Geometry: final body of the model. Coordinates: model frame, mm. A direction names the side the tool comes from. Coordinates: 2 decimals unless noted, no trailing zeros. Loops run counter-clockwise (first coordinate to the right, second up) from the corner with the lowest first, then second, coordinate; pieces in that order, holes last. Notation, with made-up numbers: (23.25, 86.5) - (36.25, 86.5) arc R19 ccw to (36.25, 103.5) - close; hole circle Ø4 at (8, 88). An arc over 180 degrees is marked (long way). Answer in a Markdown table with one row per item.
from build123d import *

# Parameters (mm, degrees)
BASE_FLANGE1_DEPTH         = 3.175
F_4_2_4_2_DIAMETER_HOLE1_D = 4.2
F_3_3_3_3_DIAMETER_HOLE1_D = 3.3
EDGE_FLANGE1_DEPTH         = 38.176085753
EDGE_FLANGE1_START         = 3.175
EDGE_FLANGE1_PROFILE_R     = 1.6
EDGE_FLANGE1_PROFILE_R_2   = 11.5
EDGE_FLANGE1_PROFILE_R_3   = 2.6
EDGE_FLANGE1_FLAT_DEPTH    = 3.175


# Sheet-metal steps are written as plain solids
with BuildPart() as part:
    # Sketch11 → Base-Flange1 (new body)
    with BuildSketch(Plane.XZ.offset(2.7625)):
        with BuildLine():
            Line((36.2, 21.175), (36.2, 15.175))
            ThreePointArc((36.2, 15.175), (30, 8.975), (23.8, 15.175))
            Line((23.8, 15.175), (23.8, 21.175))
            ThreePointArc((23.8, 21.175), (23.214213562, 22.589213562), (21.8, 23.175))
            Line((21.8, 23.175), (-7, 23.175))
            ThreePointArc((-7, 23.175), (-9.121320344, 22.296320344), (-10, 20.175))
            Line((-10, 20.175), (-10, 17.93389))
            ThreePointArc((-10, 17.93389), (-15, 12.93389), (-10, 7.93389))
            Line((-10, 7.93389), (-10, 7.7625))
            ThreePointArc((-10, 7.7625), (-9.121320344, 5.641179656), (-7, 4.7625))
            Line((-7, 4.7625), (67, 4.7625))
            ThreePointArc((67, 4.7625), (69.121320344, 5.641179656), (70, 7.7625))
            Line((70, 7.7625), (70, 7.93389))
            ThreePointArc((70, 7.93389), (75, 12.93389), (70, 17.93389))
            Line((70, 17.93389), (70, 20.175))
            ThreePointArc((70, 20.175), (69.121320344, 22.296320344), (67, 23.175))
            Line((67, 23.175), (38.2, 23.175))
            ThreePointArc((38.2, 23.175), (36.785786438, 22.589213562), (36.2, 21.175))
        make_face()
    extrude(amount=-BASE_FLANGE1_DEPTH)

    # Ø4.2 (4.2) Diameter Hole1 (through all)
    with Locations(Plane(origin=(0, -2.7625, 0), x_dir=(-1, 0, 0), z_dir=(0, -1, 0))):
        with Locations((-70, -12.93389), (10, -12.93389)):
            Hole(F_4_2_4_2_DIAMETER_HOLE1_D / 2)

    # Ø3.3 (3.3) Diameter Hole1 (through all)
    with Locations(Plane(origin=(0, 0.4125, 0), x_dir=(1, 0, 0), z_dir=(0, 1, 0))):
        with Locations((5, -12.93389), (55, -12.93389)):
            Hole(F_3_3_3_3_DIAMETER_HOLE1_D / 2)

    # Edge-Flange1 bend section (across the edge) → Edge-Flange1 (add)
    with BuildSketch(Plane(origin=(44.262809753, 0.4125, 3.175), x_dir=(0, 0, 1), z_dir=(-1, 0, 0))):
        with BuildLine():
            Line((-3.175, 1.5875), (0, 1.5875))
            ThreePointArc((0, 1.5875), (0.464967985, 0.464967985), (1.5875, 0))
            Line((1.5875, 0), (1.5875, -3.175))
            ThreePointArc((1.5875, -3.175), (-1.780096045, -1.780096045), (-3.175, 1.5875))
        make_face()
    extrude(amount=EDGE_FLANGE1_DEPTH)

    # Edge-Flange1 profile (on flange) → Edge-Flange1 flat (add)
    with BuildSketch(Plane(origin=(0, 0.4125, 3.175), x_dir=(-1, 0, 0), z_dir=(0, 0, -1)).offset(EDGE_FLANGE1_START)):
        with BuildLine():
            ThreePointArc((-6.086724, 42.5875), (-6.672510438, 44.001713562), (-8.086724, 44.5875))
            Line((-8.086724, 44.5875), (-42.262809753, 44.5875))
            ThreePointArc((-42.262809753, 44.5875), (-43.677023316, 44.001713562), (-44.262809753, 42.5875))
            Line((-44.262809753, 42.5875), (-44.262809753, 39.575887728))
            ThreePointArc((-44.262809753, 39.575887728), (-46.5, 34.902424049), (-44.262809753, 30.22896037))
            Line((-44.262809753, 30.22896037), (-44.262809753, 1.5875))
            Line((-44.262809753, 1.5875), (-6.086724, 1.5875))
            Line((-6.086724, 1.5875), (-6.086724, 42.5875))
        make_face()
        with Locations((-13.100505063, 10.688005063)):
            Circle(EDGE_FLANGE1_PROFILE_R, mode=Mode.SUBTRACT)
        with Locations((-23, 20.5875)):
            Circle(EDGE_FLANGE1_PROFILE_R_2, mode=Mode.SUBTRACT)
        with Locations((-32.899494937, 10.688005063)):
            Circle(EDGE_FLANGE1_PROFILE_R, mode=Mode.SUBTRACT)
        with Locations((-13.100505063, 30.486994937)):
            Circle(EDGE_FLANGE1_PROFILE_R, mode=Mode.SUBTRACT)
        with Locations((-32.899494937, 30.486994937)):
            Circle(EDGE_FLANGE1_PROFILE_R, mode=Mode.SUBTRACT)
        with Locations((-40.5, 34.902424049)):
            Circle(EDGE_FLANGE1_PROFILE_R_3, mode=Mode.SUBTRACT)
    extrude(amount=-EDGE_FLANGE1_FLAT_DEPTH)


solid = part.part
(1) Cut plane B-B on y = 21. Output: boundary loops of the cut face in (x, z) (3 decimals).
Verdict:
| item | result |
|---|---|
| outline | (6.087, 0) - (11.5, 0) - (11.5, 3.175) - (6.087, 3.175) - close; (34.5, 0) - (44.263, 0) - (44.263, 3.175) - (34.5, 3.175) - close |
(2) Access query for faces 4 (the face through (70, -1, 19)), 5 (the face through (-9.14, -1.2, 5.66)), 6 (the face through (23.8, -1, 18)). Directions: +Z, -Z, +X, -X, +Y, -Y. A direction counts if a zero-diameter tool reaches every point of the face in a straight line with its end or side. Return the directions, or none.
Verdict:
| item | result |
|---|---|
| face 4 | +Z, +X, +Y, -Y |
| face 5 | -Z, -X, +Y, -Y |
| face 6 | +Z, +Y, -Y |
(3) Cut plane C-C on x = 40.5. Output: boundary loops of the cut face in (y, z) (1 decimal), then the cut area to 3 significant figures.
Verdict:
| item | result |
|---|---|
| outline | (-2.8, 4.8) arc R4.8 ccw to (2, 0) - (32.7, 0) - (32.7, 3.2) - (2, 3.2) arc R1.6 cw to (0.4, 4.8) - (0.4, 23.2) - (-2.8, 23.2) - close; (37.9, 0) - (45, 0) - (45, 3.2) - (37.9, 3.2) - close |
| area | 194 mm² |
(4) First-contact query: pin 1 Ø5 at (x, y) = (32.9, 11.1) entering from +Z (3 decimals); pin 2 Ø2 at (y, z) = (27.5, 4) entering from +X; pin 3 Ø2.5 at (x, y) = (-3, -1.5) entering from -Z. Flat tips, straight axial feed; report the tip coordinate or a pass-through.
Verdict:
| item | result |
|---|---|
| pin 1 | stops at z = 3.175 |
| pin 2 | stops at x = 44.26 |
| pin 3 | stops at z = 4.76 |
(5) Ray query, probe 1 along X at (y, z) = (29.5, 2.5) (3 decimals); probe 2 along Y at (x, z) = (69, 8); probe 3 along Z at (x, y) = (63, 0) (1 decimal). Return the intervals inside material, ascending.
Verdict:
| item | result |
|---|---|
| probe 1 | x = 6.087 to 12.325, 13.876 to 15.254, 30.746 to 32.124, 33.675 to 44.263 |
| probe 2 | y = -2.76 to 0.41 |
| probe 3 | z = 4.8 to 23.2 |
(6) Pull-direction query (Y, two-part tool) for faces 1 (the face through (29, 0.412, 8)), 2 (the face through (27, 33, 3.175)), 3 (the face through (11.574, 11.581, 1.565)); classes: pulls with the +Y half, pulls with the -Y half, needs draft (parallel to the pull), parting line crosses it, or undercut.
Verdict:
| item | result |
|---|---|
| face 1 | pulls with the +Y half |
| face 2 | needs draft |
| face 3 | undercut |
(7) Cut plane A-A on x = 55. Output: boundary loops of the cut face in (y, z) (1 decimal), then the cut area to 3 significant figures.
Verdict:
| item | result |
|---|---|
| outline | (-2.8, 4.8) - (0.4, 4.8) - (0.4, 11.3) - (-2.8, 11.3) - close; (-2.8, 14.6) - (0.4, 14.6) - (0.4, 23.2) - (-2.8, 23.2) - close |
| area | 48.0 mm² |
(8) Cut plane D-D on x = 13.5. Output: boundary loops of the cut face in (y, z) (1 decimal), then the cut area to 3 significant figures.
Verdict:
| item | result |
|---|---|
| outline | (-2.8, 4.8) arc R4.8 ccw to (2, 0) - (9.6, 0) - (9.6, 3.2) - (2, 3.2) arc R1.6 cw to (0.4, 4.8) - (0.4, 23.2) - (-2.8, 23.2) - close; (12.6, 0) - (14.5, 0) - (14.5, 3.2) - (12.6, 3.2) - close; (27.5, 0) - (29.4, 0) - (29.4, 3.2) - (27.5, 3.2) - close; (32.4, 0) - (45, 0) - (45, 3.2) - (32.4, 3.2) - close |
| area | 150 mm² |
